Job drawing, mm, ordinate dimensions from the low corner. One solid piece. Give positions to 0.01 mm unless a question says otherwise; leave off trailing zeros. Write each loop counter-clockwise with the first axis right and the second up, starting at its lowest first coordinate (ties: lowest second). Pieces come first, ordered by that corner, then holes. Notation, with made-up numbers: (50, 56) -> (59, 56) arc R21 cw to (59, 95) -> close; hole circle Ø8 at (-24.75, -38). An arc over 180 degrees is marked (long way). One line per question, with ' | ' between items. Start each with the question number.
(1) Pin check, flat tips, straight feed: P1, Ø8, axis at x = 25.5, y = 62, coming from the +Z side; P2, Ø6.5, axis at x = 10, z = 10, coming from the -Y side; P3, Ø10.5, axis at y = 18, z = 20, coming from the -X side. Stop position of each tip, or through.
(2) Band-saw the part on A-A, the plane x = 10. Give the cut face in (y, z), and give its area (3 significant figures).
(3) Pull direction Y, two halves, no side cores. Call the marked faces 1, 2, 3 and 4: released by +Y, released by -Y, zero draft, split by the parting line, or undercut.
(4) Band-saw the part on B-B, the plane z = 10. Give the cut face in (x, y).
(5) Band-saw the part on C-C, the plane y = 50. Give the cut face in (x, z), and give its area (3 significant figures).
(6) Drill centre lines: probe 1 along Y at (x, z) = (28.45, 20); probe 2 along Z at (x, y) = (10, 72.1); probe 3 along Y at (x, z) = (13, 19). Where is each one in solid material? Low to high. Write a range as from..to.
(7) Band-saw the part on D-D, the plane x = 21.75. Give the cut face in (y, z), and give its area (3 significant figures).
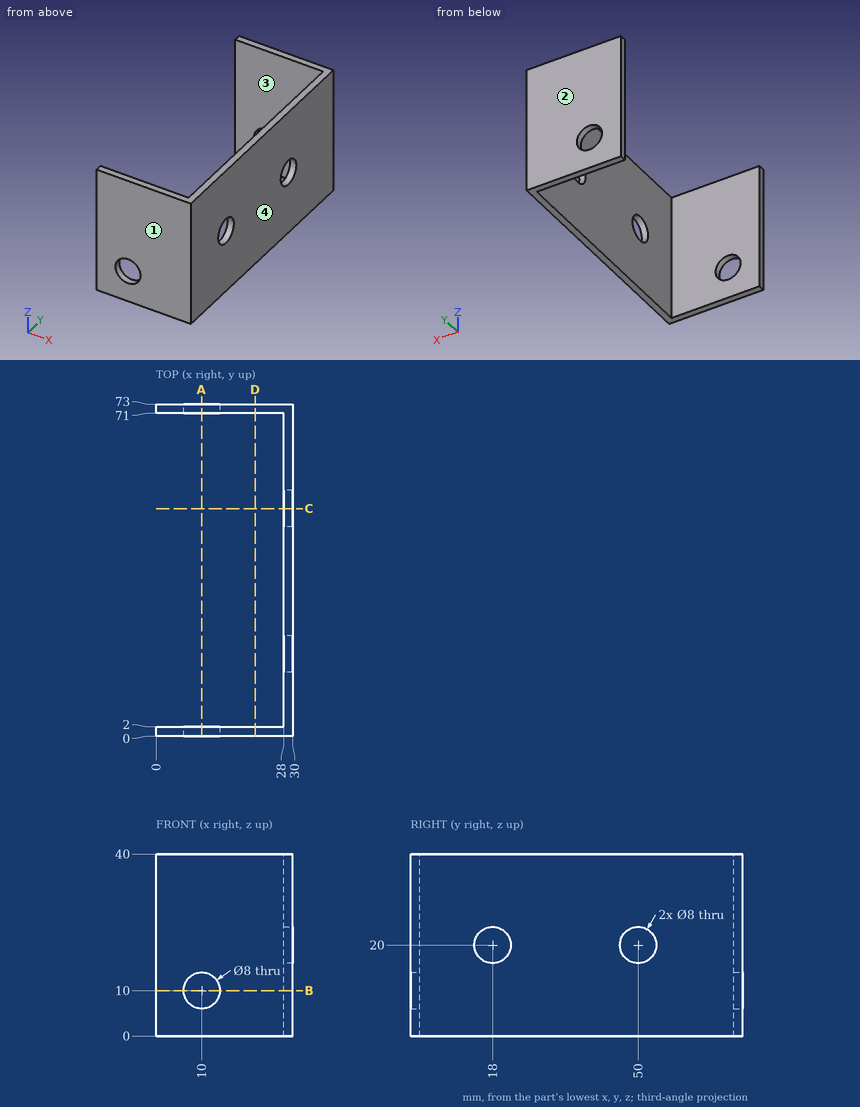
Results:
1) P1: stops at z = 40 | P2: passes through | P3: stops at x = 28
2) outline: (0, 0) -> (2, 0) -> (2, 6) -> (0, 6) -> close; (0, 14) -> (2, 14) -> (2, 40) -> (0, 40) -> close; (71, 0) -> (73, 0) -> (73, 6) -> (71, 6) -> close; (71, 14) -> (73, 14) -> (73, 40) -> (71, 40) -> close | area: 128 mm²
3) face 1: released by -Y | face 2: released by +Y | face 3: undercut | face 4: zero draft
4) outline: (0, 0) -> (6, 0) -> (6, 2) -> (0, 2) -> close; (0, 71) -> (6, 71) -> (6, 73) -> (0, 73) -> close; (14, 0) -> (30, 0) -> (30, 73) -> (14, 73) -> (14, 71) -> (28, 71) -> (28, 2) -> (14, 2) -> close
5) outline: (28, 0) -> (30, 0) -> (30, 16) -> (28, 16) -> close; (28, 24) -> (30, 24) -> (30, 40) -> (28, 40) -> close | area: 64.0 mm²
6) probe 1: y = 0..14, 22..46, 54..73 | probe 2: z = 0..6, 14..40 | probe 3: y = 0..2, 71..73
7) outline: (0, 0) -> (2, 0) -> (2, 40) -> (0, 40) -> close; (71, 0) -> (73, 0) -> (73, 40) -> (71, 40) -> close | area: 160 mm²
